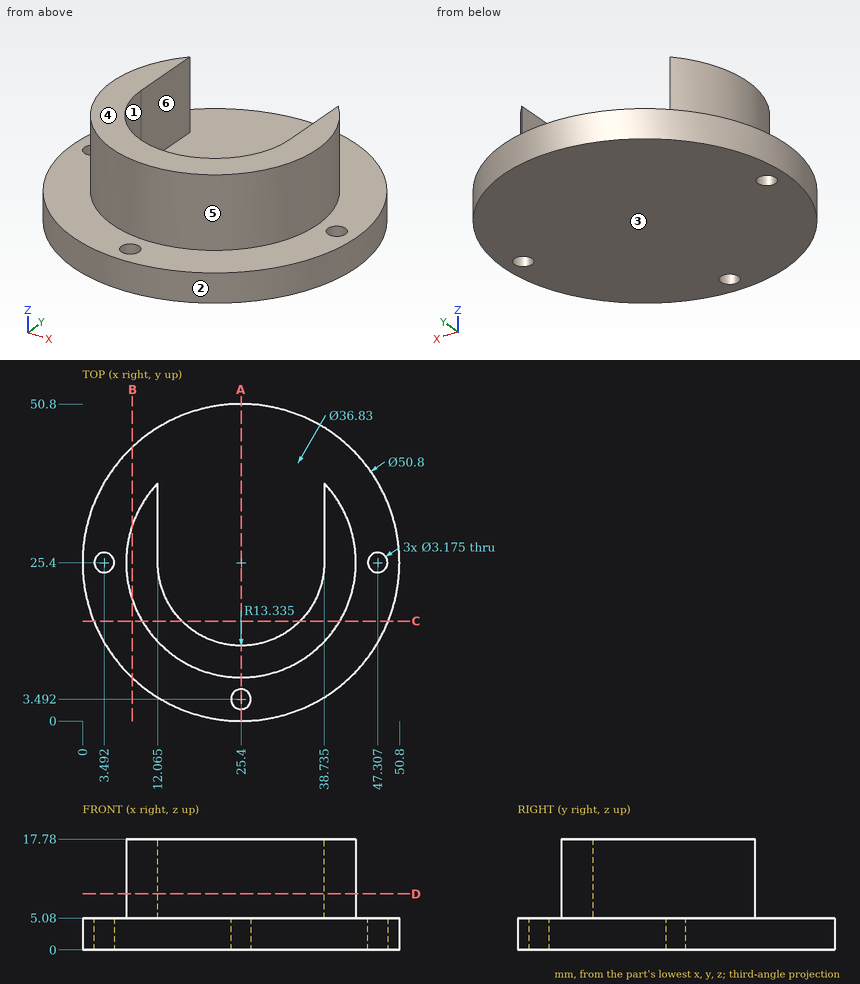
Can you work these out from the drawing? Everything is in mm from the part's minimum corner. A direction names the side the tool comes from. Round coordinates to 2 decimals unless told otherwise and drop trailing zeros. Order: outer loops, then holes, each group sorted by start corner. A loop starts at its lowest first (then second) coordinate and runs counter-clockwise, first axis right, second up. Notation, with made-up numbers: (54.25, -5.5) -> (82.25, -5.5) arc R16 cw to (82.25, 21.5) -> close; hole circle Ø5 at (2, 61.25). An arc over 180 degrees is marked (long way). Use CSV: the item, a comma, the result in double quotes.
1. I'm going to push flat-ended pins straight in: P1, Ø8, axis at x = 24.5, y = 37, coming from the +Z side; P2, Ø5, axis at x = 22.5, z = 7, coming from the -Y side; P3, Ø10, axis at y = 12.5, z = 5, coming from the -X side. Where does each tip first touch, or does it pass through?
Recorded:
P1,"stops at z = 5.08"
P2,"stops at y = 0.03"
P3,"stops at x = 1.26"
2. I want a section at D-D on z = 9. List the corners of the cut face in (x, y) for me (1 decimal), and give its area (3 significant figures).
Recorded:
outline,"(12.1, 25.4) -> (12.1, 38.1) arc R18.4 ccw (long way) to (38.7, 38.1) -> (38.7, 25.4) arc R13.3 cw to start"
area,"342 mm2"
3. I want a section at C-C on y = 16. List the corners of the cut face in (x, z) for me (1 decimal).
Recorded:
outline,"(1.8, 0) -> (49, 0) -> (49, 5.1) -> (41.2, 5.1) -> (41.2, 17.8) -> (34.9, 17.8) -> (34.9, 5.1) -> (15.9, 5.1) -> (15.9, 17.8) -> (9.6, 17.8) -> (9.6, 5.1) -> (1.8, 5.1) -> close"
4. I need wall thicknesses on line 1 along Y through (x, z) = (25.4, 2.85) (1 decimal); line 2 along X through (y, z) = (20, 11.75) (1 decimal); line 3 along Z through (x, y) = (13.5, 8). Which ranges of each line are inside material? Lowest first, please.
Recorded:
line 1,"y = 0 to 1.9, 5.1 to 50.8"
line 2,"x = 7.8 to 13.2, 37.6 to 43"
line 3,"z = 0 to 5.08"
5. Thinking about a two-plate mould opening in X: for the marked faces 1, 2 and 3, which applies, pulls with the +X half, pulls with the -X half, needs draft (parallel to the pull), parting line crosses it, or undercut?
Recorded:
face 1,"undercut"
face 2,"parting line crosses it"
face 3,"needs draft"
6. I want a section at B-B on x = 8. List the corners of the cut face in (y, z) for me (1 decimal).
Recorded:
outline,"(6.9, 0) -> (43.9, 0) -> (43.9, 5.1) -> (31.4, 5.1) -> (31.4, 17.8) -> (19.4, 17.8) -> (19.4, 5.1) -> (6.9, 5.1) -> close"
7. Which directions (+Z, -Z, +X, -X, +Y, -Y) give clear straight access to the entire face, cutting with the end or side of a thin tool? Please do the marked faces 4, 5 and 6.
Recorded:
face 4,"+Z, +X, -X, +Y, -Y"
face 5,"+Z"
face 6,"+Z, +Y"
8. I want a section at A-A on x = 25.4. List the corners of the cut face in (y, z) for me (1 decimal).
Recorded:
outline,"(0, 0) -> (1.9, 0) -> (1.9, 5.1) -> (0, 5.1) -> close; (5.1, 0) -> (50.8, 0) -> (50.8, 5.1) -> (12.1, 5.1) -> (12.1, 17.8) -> (7, 17.8) -> (7, 5.1) -> (5.1, 5.1) -> close"
